from build123d import *

# Parameters (mm, degrees)
CROQUIS2_W              = 1
CROQUIS2_H              = 352
SALIENTE_EXTRUIR2_DEPTH = 25
CROQUIS5_R              = 1.5
CROQUIS5_R_2            = 5
CORTAR_EXTRUIR2_DEPTH   = 1
SALIENTE_EXTRUIR3_DEPTH = 1


with BuildPart() as part:
    # Croquis2 → Saliente-Extruir2 (new body)
    with BuildSketch(Plane.XY):
        with Locations((-55.840004841, -113.819624774)):
            Rectangle(CROQUIS2_W, CROQUIS2_H)
    extrude(amount=SALIENTE_EXTRUIR2_DEPTH)

    # Croquis5 → Cortar-Extruir2 (cut)
    with BuildSketch(Plane(origin=(-55.340004841, 0, 0), x_dir=(0, 0, -1), z_dir=(1, 0, 0))):
        with Locations((-12.5, 48.180375226)):
            Circle(CROQUIS5_R)
        with Locations((-12.5, -275.819624774)):
            Circle(CROQUIS5_R)
        with Locations((-12.5, -159.819624774)):
            Circle(CROQUIS5_R_2)
    extrude(amount=-CORTAR_EXTRUIR2_DEPTH, mode=Mode.SUBTRACT)

    # Croquis1 → Saliente-Extruir3 (add)
    with BuildSketch(Plane.XY):
        Polygon((-56.340004841, 62.180375226), (-61.340004841, 62.180375226), (-61.340004841, 56.180375226), (-80.340004841, 56.180375226), (-80.340004841, -13.819624774), (-61.340004841, -13.819624774), (-61.340004841, -213.819624774), (-80.340004841, -213.819624774), (-80.340004841, -283.819624774), (-61.340004841, -283.819624774), (-61.340004841, -289.819624774), (-56.340004841, -289.819624774), align=None)
    extrude(amount=SALIENTE_EXTRUIR3_DEPTH)


solid = part.part
Geometry: final body of the model. Coordinates: model frame, mm. A direction names the side the tool comes from. Coordinates: 2 decimals unless noted, no trailing zeros. Order: outer loops, then holes, each group sorted by start corner. A loop starts at its lowest first (then second) coordinate and runs counter-clockwise, first axis right, second up.
(1) First-contact query: pin 1 (7 mm diameter, centred on y = -43.5, z = 8.5, fed in from -X); pin 2 (0.5 mm diameter, centred on x = -73, z = 0.5, fed in from +Y); pin 3 (0.5 mm diameter, centred on y = -145, z = 0.5, fed in from -X). Flat tips, straight axial feed; report the tip coordinate or a pass-through.
(2) Access query for faces 1 (the face through (-56, -289.82, 11)), 2 (the face through (-56.34, -116, 13)). Directions: +Z, -Z, +X, -X, +Y, -Y. A direction counts if a zero-diameter tool reaches every point of the face in a straight line with its end or side. Return the directions, or none.
(3) Section query A-A (x = -67.5). Return the cut outline in (y, z).
(4) Material intervals for probe 1 along Y at (x, z) = (-55.55, 12.5); probe 2 along Z at (x, y) = (-77.75, -1); probe 3 along X at (y, z) = (-175.5, 21.75), sorted ascending.
(5) Section query D-D (y = -111.5). Return the cut outline in (x, z), plus the area to 3 significant figures.
(6) Section query B-B (y = -224). Return the cut outline in (x, z).
(7) Section query C-C (z = 21.5). Return the cut outline in (x, y).
(8) Draft query along Y for faces 3 (the face through (-56, 62.18, 11)), 4 (the face through (-55.833, -154.862, 13.151)), 5 (the face through (-60, -111, 0)). Return one class per face: pulls with the +Y half, pulls with the -Y half, needs draft (parallel to the pull), parting line crosses it, or undercut.
Solution:
1. pin 1: stops at x = -56.34
1. pin 2: stops at y = 56.18
1. pin 3: stops at x = -61.34
2. face 1: +Z, -Z, +X, -X, -Y
2. face 2: +Z, -X, +Y, -Y
3. outline: (-283.82, 0) - (-213.82, 0) - (-213.82, 1) - (-283.82, 1) - close; (-13.82, 0) - (56.18, 0) - (56.18, 1) - (-13.82, 1) - close
4. probe 1: y = -289.82 to -277.32, -274.32 to -164.82, -154.82 to 46.68, 49.68 to 62.18
4. probe 2: z = 0 to 1
4. probe 3: x = -56.34 to -55.34
5. outline: (-61.34, 0) - (-55.34, 0) - (-55.34, 25) - (-56.34, 25) - (-56.34, 1) - (-61.34, 1) - close
5. area: 30.0 mm2
6. outline: (-80.34, 0) - (-55.34, 0) - (-55.34, 25) - (-56.34, 25) - (-56.34, 1) - (-80.34, 1) - close
7. outline: (-56.34, -289.82) - (-55.34, -289.82) - (-55.34, 62.18) - (-56.34, 62.18) - close
8. face 3: pulls with the +Y half
8. face 4: undercut
8. face 5: needs draft
